Input: part model. Units: mm. Frame: model coordinates. A direction names the side the tool comes from. Coordinates: 2 decimals unless noted, no trailing zeros. Loops run counter-clockwise (first coordinate to the right, second up) from the corner with the lowest first, then second, coordinate; pieces in that order, holes last.
```python
from build123d import *

# Parameters (mm, degrees)
F0_R     = 11.5
F0_R_2   = 1.3
F0_R_3   = 3.5
F1_DEPTH = 4.35
F4_DEPTH = 3
F6_R     = 2.25
F7_DEPTH = 2.6
F8_R     = 1
F9_DEPTH = 8


with BuildPart() as f1:
    # F0 (on Top) → F1 (new body)
    with BuildSketch(Plane.XY):
        Circle(F0_R)
        with Locations((0, -7.95)):
            Circle(F0_R_2, mode=Mode.SUBTRACT)
        with Locations((-6.2, 0)):
            Circle(F0_R_2, mode=Mode.SUBTRACT)
        Circle(F0_R_3, mode=Mode.SUBTRACT)
        with Locations((6.2, 0)):
            Circle(F0_R_2, mode=Mode.SUBTRACT)
        with Locations((0, 7.95)):
            Circle(F0_R_2, mode=Mode.SUBTRACT)
    extrude(amount=F1_DEPTH)

    # F3 (on offset) → F4 (join)
    with BuildSketch(Plane.XY.offset(4.35)):
        with BuildLine():
            ThreePointArc((5.69221, -3.358757), (3.358757, -3.358757), (3.358757, -5.69221))
            Line((3.358757, -5.69221), (5.621499, -7.954951))
            ThreePointArc((5.621499, -7.954951), (7.954951, -7.954951), (7.954951, -5.621499))
            Line((7.954951, -5.621499), (5.69221, -3.358757))
        make_face()
        with BuildLine():
            ThreePointArc((3.358757, 5.69221), (3.358757, 3.358757), (5.69221, 3.358757))
            Line((5.69221, 3.358757), (7.954951, 5.621499))
            ThreePointArc((7.954951, 5.621499), (7.954951, 7.954951), (5.621499, 7.954951))
            Line((5.621499, 7.954951), (3.358757, 5.69221))
        make_face()
        with BuildLine():
            ThreePointArc((-5.69221, 3.358757), (-3.358757, 3.358757), (-3.358757, 5.69221))
            Line((-3.358757, 5.69221), (-5.621499, 7.954951))
            ThreePointArc((-5.621499, 7.954951), (-7.954951, 7.954951), (-7.954951, 5.621499))
            Line((-7.954951, 5.621499), (-5.69221, 3.358757))
        make_face()
        with BuildLine():
            ThreePointArc((-3.358757, -5.69221), (-3.358757, -3.358757), (-5.69221, -3.358757))
            Line((-5.69221, -3.358757), (-7.954951, -5.621499))
            ThreePointArc((-7.954951, -5.621499), (-7.954951, -7.954951), (-5.621499, -7.954951))
            Line((-5.621499, -7.954951), (-3.358757, -5.69221))
        make_face()
    extrude(amount=F4_DEPTH)

    # F6 (on offset) → F7 (cut)
    with BuildSketch(Plane.XY.offset(1.8)):
        with Locations((0, -7.95)):
            Circle(F6_R)
        with Locations((6.2, 0)):
            Circle(F6_R)
        with Locations((0, 7.95)):
            Circle(F6_R)
        with Locations((-6.2, 0)):
            Circle(F6_R)
    extrude(amount=F7_DEPTH, mode=Mode.SUBTRACT)

    # F8 (on Top) → F9 (cut)
    with BuildSketch(Plane.XY):
        with Locations((5.656854, -5.656854)):
            Circle(F8_R)
        with Locations((5.656854, 5.656854)):
            Circle(F8_R)
        with Locations((-5.656854, 5.656854)):
            Circle(F8_R)
        with Locations((-5.656854, -5.656854)):
            Circle(F8_R)
    extrude(amount=F9_DEPTH, mode=Mode.SUBTRACT)


solid = f1.part
```
Item 1: Section query A-A (x = 0). Output: boundary loops of the cut face in (y, z), then the cut area to 3 significant figures.
Result:
outline: (-11.5, 0) - (-9.25, 0) - (-9.25, 1.8) - (-10.2, 1.8) - (-10.2, 4.35) - (-11.5, 4.35) - close; (-6.65, 0) - (-3.5, 0) - (-3.5, 4.35) - (-5.7, 4.35) - (-5.7, 1.8) - (-6.65, 1.8) - close; (3.5, 0) - (6.65, 0) - (6.65, 1.8) - (5.7, 1.8) - (5.7, 4.35) - (3.5, 4.35) - close; (9.25, 0) - (11.5, 0) - (11.5, 4.35) - (10.2, 4.35) - (10.2, 1.8) - (9.25, 1.8) - close
area: 37.3 mm2
Item 2: Contact query for flat-ended pins moving along their axis: P1, Ø1.6, axis at x = 5.66, y = 5.66, coming from the -Z side; P2, Ø2, axis at x = -9, z = 1, coming from the -Y side; P3, Ø4, axis at x = 0, y = -7.95, coming from the +Z side; P4, Ø5, axis at x = 7, y = -0.5, coming from the +Z side. Output: stop coordinate, or through.
Result:
P1: passes through
P2: stops at y = -8.26
P3: stops at z = 1.8
P4: stops at z = 4.35
Item 3: Section query C-C (y = 0). Output: boundary loops of the cut face in (x, z).
Result:
outline: (-11.5, 0) - (-7.5, 0) - (-7.5, 1.8) - (-8.45, 1.8) - (-8.45, 4.35) - (-11.5, 4.35) - close; (-4.9, 0) - (-3.5, 0) - (-3.5, 4.35) - (-3.95, 4.35) - (-3.95, 1.8) - (-4.9, 1.8) - close; (3.5, 0) - (4.9, 0) - (4.9, 1.8) - (3.95, 1.8) - (3.95, 4.35) - (3.5, 4.35) - close; (7.5, 0) - (11.5, 0) - (11.5, 4.35) - (8.45, 4.35) - (8.45, 1.8) - (7.5, 1.8) - close
Item 4: Section query D-D (y = -6.25). Output: boundary loops of the cut face in (x, z).
Result:
outline: (-9.65, 0) - (-6.46, 0) - (-6.46, 7.35) - (-8.35, 7.35) - (-8.35, 4.35) - (-9.65, 4.35) - close; (-4.85, 0) - (4.85, 0) - (4.85, 7.35) - (3.92, 7.35) - (3.92, 4.35) - (1.47, 4.35) - (1.47, 1.8) - (-1.47, 1.8) - (-1.47, 4.35) - (-3.92, 4.35) - (-3.92, 7.35) - (-4.85, 7.35) - close; (6.46, 0) - (9.65, 0) - (9.65, 4.35) - (8.35, 4.35) - (8.35, 7.35) - (6.46, 7.35) - close
Item 5: Mould query, pull axis X, two halves, no side actions, for faces 4 (the face through (-1.5, 11.4, 2.1)), 5 (the face through (-6.808, -4.474, 5.829)), 6 (the face through (-4.474, 6.808, 5.829)). Classes: +X half, -X half, draft (parallel to the pull), parting line (faces both ways), or undercut.
Result:
face 4: parting line
face 5: -X half
face 6: undercut
Item 6: Line query: L1, parallel to Y at x = 0, z = 0.95; L2, parallel to X at y = 1, z = 1.75; L3, parallel to X at y = -4.75, z = 0.75. Output: solid intervals per line, ascending.
Result:
L1: y = -11.5 to -9.25, -6.65 to -3.5, 3.5 to 6.65, 9.25 to 11.5
L2: x = -11.46 to -7.03, -5.37 to -3.35, 3.35 to 5.37, 7.03 to 11.46
L3: x = -10.47 to -6.08, -5.24 to 5.24, 6.08 to 10.47
Item 7: Reachability of faces 1 (the face through (4.506, 6.839, 5.829)), 2 (the face through (-7.93, 7.98, 5.83)), 3 (the face through (-4.506, -6.839, 5.829)) from +Z, -Z, +X, -X, +Y, -Y: full face, straight path, thin tool, end or side. Return the list, or none.
Result:
face 1: +Z, +Y
face 2: +Z
face 3: +Z, -Y
